Design review of the part built by this model. Coordinates are the model's own, in mm. Coordinates: 2 decimals unless noted, no trailing zeros. Write each loop counter-clockwise with the first axis right and the second up, starting at its lowest first coordinate (ties: lowest second). Pieces come first, ordered by that corner, then holes. Notation, with made-up numbers: (57.25, 34.5) -> (75.25, 34.5) arc R32 ccw to (75.25, 72.5) -> close; hole circle Ø11 at (-3.5, 79). An arc over 180 degrees is marked (long way). One line per question, with ' | ' between items. Start each with the question number.
Q1. Add section B-B on z = 1.5. State the section outline as (x, y) points, and give its area (3 significant figures).
Q2. Wall thickness on probe 1 along X at (y, z) = (26.55, -3); probe 2 along Z at (x, y) = (0.5, 26.4); probe 3 along Z at (x, y) = (-1.5, 26.45): over which ranges is each line inside the solid? List them lowest first.
Q3. For P1, Ø1, axis at y = 27.5, z = 5.5, coming from the -X side; P2, Ø6, axis at x = 13, z = 7.5, coming from the +Y side; P3, Ø10, axis at x = 10.5, z = 1.5, coming from the +Y side, all flat-tipped, find the tip position at first contact; note any pin that passes through.
Q4. Add section C-C on x = 13. State the section outline as (y, z) points.
Q5. Add section A-A on y = 26.7. State the section outline as (x, z) points.
from build123d import *

# Parameters (mm, degrees)
BOX_W           = 60
BOX_H           = 40
BOX_DEPTH       = 60
SPHERE001_ANGLE = 180
SPHERE_ANGLE    = 180


with BuildPart() as cube:
    # Box → Box (new body)
    with BuildSketch(Plane(origin=(-30, -15, -30), x_dir=(1, 0, 0), z_dir=(0, 0, 1))):
        with Locations((30, 20)):
            Rectangle(BOX_W, BOX_H)
    extrude(amount=BOX_DEPTH)


with BuildPart() as inner:
    # Sphere001 → Sphere001 (revolve)
    with BuildSketch(Plane.XZ):
        with BuildLine():
            ThreePointArc((0, -29.7), (29.7, 0), (0, 29.7))
            Line((0, 29.7), (0, -29.7))
        make_face()
    revolve(axis=Axis((0, 0, 0), (0, 0, 1)), revolution_arc=SPHERE001_ANGLE)


with BuildPart() as cut001:
    # Sphere → Sphere (revolve)
    with BuildSketch(Plane.XZ):
        with BuildLine():
            ThreePointArc((0, -30), (30, 0), (0, 30))
            Line((0, 30), (0, -30))
        make_face()
    revolve(axis=Axis((0, 0, 0), (0, 0, 1)), revolution_arc=SPHERE_ANGLE)

    # Cut: cut Inner
    add(inner.part, mode=Mode.SUBTRACT)

    # Cut001: cut Cube
    add(cube.part, mode=Mode.SUBTRACT)


solid = cut001.part
Output values:
1) outline: (-16.52, 25) -> (-15.96, 25) arc R29.66 cw to (15.96, 25) -> (16.52, 25) arc R29.96 ccw to start | area: 10.3 mm2
2) probe 1: x = -13.64 to -12.97, 12.97 to 13.64 | probe 2: z = -14.24 to -13.6, 13.6 to 14.24 | probe 3: z = -14.08 to -13.43, 13.43 to 14.08
3) P1: stops at x = -11.89 | P2: stops at y = 27.49 | P3: stops at y = 29.47
4) outline: (25, -10.3) arc R27.04 ccw to (25, 10.3) -> (25, 9.39) arc R26.7 cw to (25, -9.39) -> close
5) outline: circle Ø27.36 at (0, 0); hole circle Ø26.02 at (0, 0)
